Autodesk Inventor part; units mm, degrees
ref_plane "YZ Plane" through (0, 0, 0) normal (1, 0, 0) x (0, 1, 0)
ref_plane "XZ Plane" through (0, 0, 0) normal (0, 1, 0) x (-1, 0, 0)
ref_plane "XY Plane" through (0, 0, 0) normal (0, 0, 1) x (1, 0, 0)
sketch "Sketch1" plane through (0, 0, 0) normal (0, 0, 1) x (1, 0, 0)
  line L0 (0, 0) -> (0, 10)
  line L1 (0, 10) -> (0, 78.5)
  line L2 (0, 78.5) -> (0, 84.5)
  line L3 (0, 84.5) -> (10, 84.5)
  line L4 (10, 84.5) -> (16, 84.5)
  line L5 (16, 84.5) -> (16, 16)
  line L6 (16, 16) -> (84.5, 16)
  line L7 (84.5, 0) -> (0, 0)
  line L8 (10, 84.5) -> (10, 10)
  line L9 (84.5, 16) -> (84.5, 10)
  line L10 (84.5, 10) -> (84.5, 0)
  line L11 (84.5, 0) -> (0, 0)
  line L12 (84.5, 10) -> (10, 10)
  circle A0 centre (13, 79.9) radius 1.25
  circle A1 centre (13, 63.4) radius 1.25
  line L13 (13, 82.5899) -> (13, 13)
  circle A2 centre (63.4, 13) radius 1.25
  circle A3 centre (79.9, 13) radius 1.25
  point P0 (13, 84.5)
  dimension "d0" = 68.5
  dimension "d1" = 10
  dimension "d2" = 10
  dimension "d3" = 6
  dimension "d6" = 10
  dimension "d7" = 6
  dimension "d8" = 0
  dimension "d9" = 2.5
  dimension "d11" = 6
  dimension "d13" = 69.9
  dimension "d14" = 2.5
  dimension "d15" = 53.4
  dimension "d16" = 0
  dimension "d17" = 84.5
  dimension "d20" = 90
extrude "Extrusion1" add sketch "Sketch1" along normal blind 3.875
sketch "Sketch2" plane through (0, 0, 3.875) normal (0, 0, 1) x (1, 0, 0)
  line L0 (0, 0) -> (84.5, 0)
  line L1 (84.5, 0) -> (84.5, 16)
  line L2 (84.5, 16) -> (16, 16)
  line L3 (16, 16) -> (16, 84.5)
  line L4 (16, 84.5) -> (0, 84.5)
  line L5 (0, 84.5) -> (0, 0)
  circle A0 centre (13, 63.4) radius 1.25
  circle A1 centre (13, 79.9) radius 1.25
  circle A2 centre (63.4, 13) radius 1.25
  circle A3 centre (79.9, 13) radius 1.25
  line L6 (0, 0) -> (5.4402, 0)
  line L7 (10, 10) -> (10, 84.5)
  line L8 (10, 84.5) -> (0, 84.5)
  line L9 (0, 84.5) -> (0, 0)
  line L10 (84.5, 0) -> (84.5, 16)
  line L11 (0, 0) -> (84.5, 0)
  line L12 (84.5, 0) -> (84.5, 10)
  line L13 (84.5, 10) -> (10, 10)
  line L14 (0, 5.0322) -> (0, 0)
  dimension "d24" = 10
  dimension "d25" = 10
extrude "Extrusion2" add sketch "Sketch2" along normal blind 2.25 contours L5 L4 L7 L13 L1 L0
sketch "Sketch5" plane through (0, 0, 6.125) normal (0, 0, 1) x (1, 0, 0)
  line L0 (10, 10) -> (10, 84.5)
  line L1 (10, 84.5) -> (0, 84.5)
  line L2 (0, 84.5) -> (0, 0)
  line L3 (0, 0) -> (84.5, 0)
  line L4 (84.5, 0) -> (84.5, 10)
  line L5 (84.5, 10) -> (10, 10)
  circle A0 centre (79.9, 13) radius 1.25
  circle A1 centre (63.4, 13) radius 1.25
  circle A2 centre (13, 79.9) radius 1.25
  circle A3 centre (13, 63.4) radius 1.25
  line L6 (10, 84.5) -> (10, 10)
  line L7 (10, 10) -> (84.5, 10)
  line L8 (84.5, 10) -> (84.5, 16)
  line L9 (84.5, 16) -> (16, 16)
  line L10 (16, 16) -> (16, 84.5)
  line L11 (16, 84.5) -> (10, 84.5)
  line L12 (0, 84.5) -> (16, 84.5)
  line L13 (16, 0) -> (0, 0)
  line L14 (0, 0) -> (0, 84.5)
  line L15 (0, 0) -> (84.5, 0)
  line L16 (84.5, 0) -> (84.5, 16)
  line L17 (84.5, 16) -> (16, 16)
  line L18 (0, 16) -> (0, 0)
  line L19 (16, 84.5) -> (16, 16)
extrude "Extrusion5" add sketch "Sketch5" along normal blind 3.875 contours L5 L4 L3 L2 L1 L0 | L0 L11 L10 L9 L8 L5 | A0 | A1 | A2 | A3
sketch "Sketch6" plane through (0, 0, 0) normal (-1, 0, 0) x (0, 0, 1)
  line L0 (3.875, 84.5) -> (3.875, 10)
  line L1 (3.875, 84.5) -> (6.125, 84.5)
  line L2 (6.125, 10) -> (6.125, 84.5)
  line L3 (3.875, 10) -> (6.125, 10)
  line L4 (0, 84.5) -> (10, 84.5)
  line L5 (0, 84.5) -> (0, 0)
  line L6 (0, 0) -> (10, 0)
  line L7 (10, 84.5) -> (10, 0)
  circle A0 centre (5, 44.25) radius 2
  circle A1 centre (5, 34) radius 2
  point P0 (6.125, 47.25)
  dimension "d51" = 4
  dimension "d52" = 4
  dimension "d53" = 10
  dimension "d54" = 5
  dimension "d55" = 5
  dimension "d73" = 24
  dimension "d74" = 34.25
extrude "Extrusion6" cut sketch "Sketch6" against normal blind 10 contours A0 L2 L0 | L0 A0 | A0 L2 | A1 L2 L0 | L0 A1 | A1 L2
sketch "Sketch7" plane through (0, 0, 0) normal (0, -1, 0) x (1, 0, 0)
  line L0 (10, 3.875) -> (84.5, 3.875)
  line L1 (10, 3.875) -> (10, 6.125)
  line L2 (84.5, 6.125) -> (10, 6.125)
  line L3 (84.5, 3.875) -> (84.5, 6.125)
  line L4 (0, 0) -> (0, 10)
  line L5 (0, 0) -> (84.5, 0)
  line L6 (84.5, 0) -> (84.5, 10)
  line L7 (0, 10) -> (84.5, 10)
  circle A0 centre (44.25, 5) radius 2
  circle A1 centre (38, 5) radius 2
  point P0 (84.5, 5)
  dimension "d60" = 4
  dimension "d61" = 4
  dimension "d62" = 10
  dimension "d63" = 5
  dimension "d64" = 5
  dimension "d77" = 28
  dimension "d78" = 34.25
extrude "Extrusion7" cut sketch "Sketch7" against normal blind 10 contours A1 L2 L0 | L0 A1 | A1 L2 | A0 L2 L0 | L0 A0 | A0 L2
sketch "Sketch8" plane through (0, 0, 0) normal (0, 0, -1) x (-1, 0, 0)
  line L0 (0, 0) -> (-84.5, 0)
  line L1 (0, 84.5) -> (0, 0)
  line L2 (-16, 84.5) -> (0, 84.5)
  line L3 (-16, 16) -> (-16, 84.5)
  line L4 (-84.5, 16) -> (-16, 16)
  line L5 (-84.5, 0) -> (-84.5, 16)
  circle A0 centre (-13, 63.4) radius 1.25
  circle A1 centre (-13, 79.9) radius 1.25
  circle A2 centre (-63.4, 13) radius 1.25
  circle A3 centre (-79.9, 13) radius 1.25
  circle A4 centre (-79.9, 13) radius 1.25
  circle A5 centre (-63.4, 13) radius 1.25
  circle A6 centre (-13, 63.4) radius 1.25
  circle A7 centre (-13, 79.9) radius 1.25
extrude "Extrusion8" cut sketch "Sketch8" against normal through all contours A0 | A1 | A2 | A3
equation "\"d0\" = PCB_L"
equation "\"d1\" = Clamp_Bracket_W"
equation "\"d2\" = Clamp_Bracket_W"
equation "\"d3\" = Trim_Mount_W"
equation "\"d6\" = d1"
equation "\"d7\" = d3"
equation "\"d11\" = Trim_Mount_W"
equation "\"d14\" = d9"
equation "\"d17\" = d0 + d1 + d11"
equation "\"d22\" = Mount_W_Back"
equation "\"d24\" = Clamp_Bracket_W"
equation "\"d25\" = Clamp_Bracket_W"
equation "\"d49\" = Mount_W_Front"
equation "\"d51\" = Post_Mount_Hole_D"
equation "\"d52\" = d51"
equation "\"d54\" = 0.5 * d53"
equation "\"d55\" = 0.5 * d53"
equation "\"d73\" = 0.5 * PCB_W - PCB_W_Offset"
equation "\"d74\" = 0.5 * PCB_L"
equation "\"d58\" = Clamp_Bracket_W"
equation "\"d60\" = d51"
equation "\"d61\" = d51"
equation "\"d63\" = 0.5 * d62"
equation "\"d64\" = 0.5 * d62"
equation "\"d77\" = 0.5 * PCB_W + PCB_W_Offset"
equation "\"d78\" = 0.5 * PCB_L"
equation "\"d67\" = Clamp_Bracket_W"
properties part number "UCD V1.0 PCB Holder"
The listing builds one solid part. Answer for the finished solid, in the listing's coordinates (mm). A direction names the side the tool comes from. Give positions to 0.01 mm unless a question says otherwise; leave off trailing zeros. Write each loop counter-clockwise with the first axis right and the second up, starting at its lowest first coordinate (ties: lowest second). Pieces come first, ordered by that corner, then holes. Notation, with made-up numbers: (-1, 11.25) -> (21, 11.25) arc R17 ccw to (21, 31.25) -> close; hole circle Ø8 at (60.5, -27). An arc over 180 degrees is marked (long way). One line per question, with ' | ' between items. Start each with the question number.
1. Given pin 1 Ø1.8 at (x, z) = (41, 5) entering from +Y; pin 2 Ø2 at (x, y) = (79.9, 13) entering from -Z; pin 3 Ø5 at (x, z) = (38, 5) entering from +Y; pin 4 Ø1.5 at (y, z) = (22, 7) entering from +X, each flat-ended and moving along its own axis, determine where each tip first touches the part or whether it passes through.
2. Section A-A (x = 44.25) is taken. Determine the outline of the cut face in (y, z) (3 decimals).
3. For a pull along Y with two mould halves and no side action, classify faces 4 (the cylindrical face through (12.423, 78.791, 8.035)), 5 (the flat face through (65, 10, 5)), 6 (the flat face through (84.5, 8, 5)) as pulls with the +Y half, pulls with the -Y half, needs draft (parallel to the pull), parting line crosses it, or undercut.
4. Find the intervals of material crossed by probe 1 along X at (y, z) = (4, 5); probe 2 along Y at (x, z) = (13, 9.2); probe 3 along Y at (x, z) = (5, 6.75), in increasing order.
5. Section D-D (x = 63.4) is taken. Determine the outline of the cut face in (y, z) (3 decimals), plus the area to 3 significant figures.
6. For faces 1 (the flat face through (10, 65, 5)), 2 (the flat face through (16, 50, 8)), 3 (the cylindrical face through (5, 32, 5)), determine the directions among +Z, -Z, +X, -X, +Y, -Y from which every point of the face is accessible in a straight line to the end or side of a thin tool.
7. Section C-C (z = 5) is taken. Determine the outline of the cut face in (x, y), plus the area to 3 significant figures.
8. Section B-B (y = 13) is taken. Determine the outline of the cut face in (x, z) (3 decimals), plus the area to 3 significant figures.
Response values:
1) pin 1: y = 10 | pin 2: through | pin 3: y = 16 | pin 4: x = 16
2) outline: (0, 0) -> (16, 0) -> (16, 3.875) -> (10, 3.875) -> (10, 3) -> (0, 3) -> close; (0, 7) -> (10, 7) -> (10, 6.125) -> (16, 6.125) -> (16, 10) -> (0, 10) -> close
3) face 4: undercut | face 5: pulls with the +Y half | face 6: needs draft
4) probe 1: 0 to 36, 40 to 42.25, 46.25 to 84.5 | probe 2: 0 to 62.15, 64.65 to 78.65, 81.15 to 84.5 | probe 3: 0 to 33.03, 34.97 to 43.28, 45.22 to 84.5
5) outline: (0, 0) -> (11.75, 0) -> (11.75, 3.875) -> (10, 3.875) -> (10, 6.125) -> (11.75, 6.125) -> (11.75, 10) -> (0, 10) -> close; (14.25, 0) -> (16, 0) -> (16, 3.875) -> (14.25, 3.875) -> close; (14.25, 6.125) -> (16, 6.125) -> (16, 10) -> (14.25, 10) -> close | area: 127 mm2
6) face 1: +X, +Y | face 2: +Z, -Z, +X, +Y | face 3: -X
7) outline: (0, 0) -> (36, 0) -> (36, 10) -> (10, 10) -> (10, 32) -> (0, 32) -> close; (0, 36) -> (10, 36) -> (10, 42.25) -> (0, 42.25) -> close; (0, 46.25) -> (10, 46.25) -> (10, 84.5) -> (0, 84.5) -> close; (40, 0) -> (42.25, 0) -> (42.25, 10) -> (40, 10) -> close; (46.25, 0) -> (84.5, 0) -> (84.5, 10) -> (46.25, 10) -> close | area: 1,430 mm2
8) outline: (0, 0) -> (62.15, 0) -> (62.15, 3.875) -> (10, 3.875) -> (10, 6.125) -> (62.15, 6.125) -> (62.15, 10) -> (0, 10) -> close; (64.65, 0) -> (78.65, 0) -> (78.65, 3.875) -> (64.65, 3.875) -> close; (64.65, 6.125) -> (78.65, 6.125) -> (78.65, 10) -> (64.65, 10) -> close; (81.15, 0) -> (84.5, 0) -> (84.5, 3.875) -> (81.15, 3.875) -> close; (81.15, 6.125) -> (84.5, 6.125) -> (84.5, 10) -> (81.15, 10) -> close | area: 639 mm2
